```python
from build123d import *

# Parameters (mm, degrees)
F0_W     = 3.1
F0_H     = 120
F1_DEPTH = 1
F0_W_2   = 10
F0_W_3   = 15
F0_H_2   = 119.9958917713
F0_W_4   = 2
F2_DEPTH = 8


with BuildPart() as f1:
    # F0 (on Top) → F1 (new body)
    with BuildSketch(Plane.XY):
        with Locations((-1.55, -15.0552866608)):
            Rectangle(F0_W, F0_H)
    extrude(amount=F1_DEPTH)



with BuildPart() as f1b:
    # F0 (on Top) → F1, piece 2 (new body)
    with BuildSketch(Plane.XY):
        with Locations((7, -15.0552866608)):
            Rectangle(F0_W_2, F0_H)
    extrude(amount=F1_DEPTH)


with BuildPart() as f1c:
    # F0 (on Top) → F1, piece 3 (new body)
    with BuildSketch(Plane.XY):
        with Locations((-12.6, -15.0552866608)):
            Rectangle(F0_W_3, F0_H)
    extrude(amount=F1_DEPTH)


with BuildPart() as f1d:
    # F0 (on Top) → F1, piece 4 (new body)
    with BuildSketch(Plane.XY):
        with Locations((26.6, -15.0532325464)):
            Rectangle(F0_W_3, F0_H_2)
    extrude(amount=F1_DEPTH)


with BuildPart() as f1e:
    # F0 (on Top) → F1, piece 5 (new body)
    with BuildSketch(Plane.XY):
        Polygon((17.1, 44.9447133392), (14, 44.9447133392), (14, -75.0468607033), (17.1, -75.0511784321), align=None)
    extrude(amount=F1_DEPTH)


with BuildPart() as f1_1:
    add(f1.part)

    add(f1b.part)  # F2 merges F1b

    add(f1c.part)  # F2 merges F1c

    add(f1d.part)  # F2 merges F1d

    add(f1e.part)  # F2 merges F1e
    # F0 (on Top) → F2 (join)
    with BuildSketch(Plane.XY):
        with Locations((-4.1, -15.0552866608)):
            Rectangle(F0_W_4, F0_H)
        with Locations((1, -15.0552866608)):
            Rectangle(F0_W_4, F0_H)
        Polygon((14, 44.9447133392), (12, 44.9447133392), (12, -75.0552866608), (14, -75.0468607033), align=None)
        with Locations((18.1, -15.0532325464)):
            Rectangle(F0_W_4, F0_H_2)
    extrude(amount=F2_DEPTH)


solid = f1_1.part
```
Geometry check sheet. Reference: the model listing, model coordinates, mm. A direction names the side the tool comes from. Give positions to 0.01 mm unless a question says otherwise; leave off trailing zeros. Write each loop counter-clockwise with the first axis right and the second up, starting at its lowest first coordinate (ties: lowest second). Pieces come first, ordered by that corner, then holes.
1) Section check B-B, the plane y = -1.5. Record the boundary of the cut face in (x, z), and give its area (3 significant figures).
2) Gauge pin test, flat ends, axial feed: pin 1 (1.6 mm diameter, centred on x = -1.5, y = -8, fed in from +Z); pin 2 (4 mm diameter, centred on x = -0.5, y = -40.5, fed in from -Z); pin 3 (3.5 mm diameter, centred on y = 15, z = 3.5, fed in from +X); pin 4 (1.5 mm diameter, centred on x = 19.5, z = 5.5, fed in from -Y). Record the tip position at first contact, or that the pin passes through.
3) Section check A-A, the plane z = 3.75. Record the boundary of the cut face in (x, y), and give its area (3 significant figures).
4) Section check C-C, the plane x = -14.5. Record the boundary of the cut face in (y, z).
5) Release check for a two-part mould opening along X. For faces 6 (the flat face through (-4, -75.055, 2)), 7 (the flat face through (19.1, -16, 4)), 8 (the flat face through (-5.1, -16, 4)), 9 (the flat face through (0, -16, 4)) record: pulls with the +X half, pulls with the -X half, needs draft (parallel to the pull), parting line crosses it, or undercut.
6) Access from +Z, -Z, +X, -X, +Y, -Y to the whole of each face (thin tool, end or side, straight path). Record for faces 1 (the flat face through (7, -14, 0)), 2 (the flat face through (-13, -14, 1)), 3 (the flat face through (18, -14, 8)), 4 (the flat face through (26, -14, 1)), 5 (the flat face through (17.1, -16, 4)).
7) Material ranges on L1, parallel to X at y = -15, z = 6.75; L2, parallel to Z at x = 10, y = 36, recorded low to high.
Computed:
1. outline: (-20.1, 0) - (34.1, 0) - (34.1, 1) - (19.1, 1) - (19.1, 8) - (17.1, 8) - (17.1, 1) - (14, 1) - (14, 8) - (12, 8) - (12, 1) - (2, 1) - (2, 8) - (0, 8) - (0, 1) - (-3.1, 1) - (-3.1, 8) - (-5.1, 8) - (-5.1, 1) - (-20.1, 1) - close
1. area: 110 mm2
2. pin 1: stops at z = 1
2. pin 2: stops at z = 0
2. pin 3: stops at x = 19.1
2. pin 4: stops at y = -75.05
3. outline: (-5.1, -75.06) - (-3.1, -75.06) - (-3.1, 44.94) - (-5.1, 44.94) - close; (0, -75.06) - (2, -75.06) - (2, 44.94) - (0, 44.94) - close; (12, -75.06) - (14, -75.05) - (14, 44.94) - (12, 44.94) - close; (17.1, -75.05) - (19.1, -75.05) - (19.1, 44.94) - (17.1, 44.94) - close
3. area: 960 mm2
4. outline: (-75.06, 0) - (44.94, 0) - (44.94, 1) - (-75.06, 1) - close
5. face 6: needs draft
5. face 7: pulls with the +X half
5. face 8: pulls with the -X half
5. face 9: undercut
6. face 1: -Z, +X, -X, +Y, -Y
6. face 2: +Z, -X, +Y, -Y
6. face 3: +Z, +X, -X, +Y, -Y
6. face 4: +Z, +X, +Y, -Y
6. face 5: +Z, +Y, -Y
7. L1: x = -5.1 to -3.1, 0 to 2, 12 to 14, 17.1 to 19.1
7. L2: z = 0 to 1
